```python
from build123d import *

# Parameters (mm, degrees)
PAD_DEPTH     = 55
PAD001_DEPTH  = 46.65
SKETCH003_W   = 5
SKETCH003_H   = 50
PAD002_DEPTH  = 46.65
PAD003_DEPTH  = 46.65
CHAMFER_ANGLE = 20
CHAMFER_SIZE  = 10


with BuildPart() as part:
    # Sketch → Pad (new body)
    with BuildSketch(Plane.XZ):
        Polygon((-23.325, 3), (-23.325, -20), (-20.325, -20), (-20.325, 0), (20.325, 0), (20.325, -35), (23.325, -35), (23.325, 3), align=None)
    extrude(amount=PAD_DEPTH)

    # Sketch001 (on Face1 of Pad) → Pad001 (join)
    with BuildSketch(Plane(origin=(-23.325, 0, 0), x_dir=(0, 0, -1), z_dir=(-1, 0, 0))):
        Polygon((-3, 39), (-3, 55), (-68, 92.527767), (-68, 76.527767), align=None)
    extrude(amount=-PAD001_DEPTH)

    # Sketch003 (on Face12 of Pad001) → Pad002 (join)
    with BuildSketch(Plane(origin=(-23.325, 0, 0), x_dir=(0, 0, -1), z_dir=(-1, 0, 0))):
        with Locations((-65.5, 101.527767)):
            Rectangle(SKETCH003_W, SKETCH003_H)
    extrude(amount=-PAD002_DEPTH)

    # Sketch004 (on DatumPlane) → Pad003 (join)
    with BuildSketch(Plane(origin=(-23.325, 0, 0), x_dir=(0, 0, -1), z_dir=(-1, 0, 0))):
        Polygon((-68, 0), (-3, 0), (-3, 39), (-68, 76.527767), align=None)
    extrude(amount=-PAD003_DEPTH)

    # Chamfer
    chamfer_edges = [part.edges().sort_by_distance(p)[0] for p in [
        (0, -126.527767, 63),
    ]]
    chamfer_side = part.faces().sort_by_distance((0, -108.084392, 63))[0]
    chamfer(chamfer_edges, length=CHAMFER_SIZE, angle=CHAMFER_ANGLE, reference=chamfer_side)


solid = part.part
```
Geometry: final body of the model. Coordinates: model frame, mm. A direction names the side the tool comes from. Coordinates: 2 decimals unless noted, no trailing zeros. Order: outer loops, then holes, each group sorted by start corner. A loop starts at its lowest first (then second) coordinate and runs counter-clockwise, first axis right, second up. Notation, with made-up numbers: (72.25, -8.75) -> (113.25, -8.75) arc R9 cw to (113.25, 1.25) -> close; hole circle Ø10 at (-38.75, 71.5). An arc over 180 degrees is marked (long way). Answer in a Markdown table with one row per item.
Item 1: Draft query along X for faces 6 (the flat face through (22, -27, -35)), 7 (the flat face through (-23.325, -36, 34)), 8 (the flat face through (20.325, -27, -17)). Return one class per face: released by +X, released by -X, zero draft, split by the parting line, or undercut.
Return value:
| item | result |
|---|---|
| face 6 | zero draft |
| face 7 | released by -X |
| face 8 | undercut |
Item 2: Ray query, L1, parallel to X at y = -22, z = -4 (3 decimals); L2, parallel to Z at x = 19.5, y = -8; L3, parallel to Z at x = 19.5, y = -114.5. Return the intervals inside material, ascending.
Return value:
| item | result |
|---|---|
| L1 | x = -23.325 to -20.325, 20.325 to 23.325 |
| L2 | z = 0 to 68 |
| L3 | z = 63 to 68 |
Item 3: Section D-D on z = 25. Output: boundary loops of the cut face in (x, y) (3 decimals).
Return value:
| item | result |
|---|---|
| outline | (-23.325, -67.702) -> (23.325, -67.702) -> (23.325, 0) -> (-23.325, 0) -> close |
Item 4: Access query for faces 1 (the flat face through (0, 0, 29)), 2 (the flat face through (-22, -27, -20)), 3 (the flat face through (-20.325, -27, -10)), 4 (the flat face through (23.325, -36, 17)), 5 (the flat face through (3, -55, 1)). Directions: +Z, -Z, +X, -X, +Y, -Y. A direction counts if a zero-diameter tool reaches every point of the face in a straight line with its end or side. Return the directions, or none.
Return value:
| item | result |
|---|---|
| face 1 | +Z, -Z, +X, -X, +Y |
| face 2 | -Z, -X, +Y, -Y |
| face 3 | -Z, +Y, -Y |
| face 4 | +Z, -Z, +X, +Y, -Y |
| face 5 | -Z, +X, -X, -Y |
Item 5: Contact query for flat-ended pins moving along their axis: P1, Ø0.9, axis at x = -22, y = -36.5, coming from the -Z side; P2, Ø4, axis at x = 13.5, y = -112, coming from the -Z side; P3, Ø11.5, axis at x = 5, z = -7.5, coming from the -Y side; P4, Ø3, axis at x = 17, z = 36.5, coming from the -Y side. Output: stop coordinate, or through.
Return value:
| item | result |
|---|---|
| P1 | stops at z = -20 |
| P2 | stops at z = 63 |
| P3 | passes through |
| P4 | stops at y = -75.21 |
Item 6: Section C-C on z = -22.5. Output: boundary loops of the cut face in (x, y) (3 decimals), plus the area to 3 significant figures.
Return value:
| item | result |
|---|---|
| outline | (20.325, -55) -> (23.325, -55) -> (23.325, 0) -> (20.325, 0) -> close |
| area | 165 mm² |
Item 7: Section B-B on y = -52. Output: boundary loops of the cut face in (x, z) (3 decimals), plus the area to 3 significant figures.
Return value:
| item | result |
|---|---|
| outline | (-23.325, -20) -> (-20.325, -20) -> (-20.325, 0) -> (20.325, 0) -> (20.325, -35) -> (23.325, -35) -> (23.325, 68) -> (-23.325, 68) -> close |
| area | 3,340 mm² |
Item 8: Section A-A on x = 10.5. Output: boundary loops of the cut face in (y, z).
Return value:
| item | result |
|---|---|
| outline | (-126.53, 66.64) -> (-116.53, 63) -> (-89.64, 63) -> (-55, 3) -> (-55, 0) -> (0, 0) -> (0, 68) -> (-126.53, 68) -> close |
